from build123d import *

# Parameters (mm, degrees)
SKETCH1_W           = 11.699975178
SKETCH1_H           = 11.699996949
SKETCH1_W_2         = 11.699990436
SKETCH1_H_2         = 11.699981689
SKETCH1_W_3         = 11.699990437
SKETCH1_H_3         = 11.699975177
SKETCH1_W_4         = 11.699981689
SKETCH1_H_4         = 11.699990436
BOSS_EXTRUDE1_DEPTH = 1817.878
CUT_EXTRUDE1_REACH  = 1819.878


with BuildPart() as part:
    # Sketch1 → Boss-Extrude1 (new body)
    with BuildSketch(Plane.XY):
        Polygon((22.500515052, 22.499297556), (-22.499484399, 22.499298105), (-22.499484948, -22.500701346), (-4.249491942, -22.500701568), (-4.249491942, -22.200733242), (-4.24949208, -18.000719999), (-6.799479919, -18.000719999), (-6.799480207, -9.200732353), (-4.799480391, -7.200732362), (4.800525817, -7.200732047), (6.8005258, -9.200731855), (6.800526088, -18.000720263), (4.250507877, -18.000720263), (4.250508015, -22.200733153), (4.250508015, -22.500701672), (22.500514502, -22.500701895), (22.500514725, -4.250714302), (22.200520351, -4.250714302), (18.000507108, -4.25071444), (18.000507108, -6.800702279), (9.200519462, -6.800702567), (7.200519471, -4.800702751), (7.200519156, 4.799303458), (9.200518964, 6.79930344), (18.000507424, 6.799303729), (18.000507424, 4.249285514), (22.200520261, 4.249285652), (22.500514829, 4.249285652), align=None)
        with BuildLine():
            Line((-4.249491247, 17.999291576), (-4.249490956, 22.199304807))
            Line((-4.249490956, 22.199304807), (-3.949472548, 22.199304807))
            Line((-3.949472548, 22.199304807), (-3.481695222, 21.73152644))
            ThreePointArc((-3.481695222, 21.73152644), (-2.670636178, 21.189593132), (-1.713926324, 20.999291428))
            Line((-1.713926324, 20.999291428), (1.714975167, 20.999291428))
            ThreePointArc((1.714975167, 20.999291428), (2.671722509, 21.189608628), (3.482801459, 21.731583767))
            Line((3.482801459, 21.731583767), (3.950490798, 22.199304487))
            Line((3.950490798, 22.199304487), (4.250509108, 22.199304487))
            Line((4.250509108, 22.199304487), (4.250508817, 17.999291575))
            Line((4.250508817, 17.999291575), (6.800527063, 17.999291575))
            Line((6.800527063, 17.999291575), (6.800526453, 9.199302988))
            Line((6.800526453, 9.199302988), (4.800526064, 7.199302969))
            Line((4.800526064, 7.199302969), (-4.799479817, 7.199303635))
            Line((-4.799479817, 7.199303635), (-6.799479854, 9.199304042))
            Line((-6.799479854, 9.199304042), (-6.799479244, 17.999291576))
            Line((-6.799479244, 17.999291576), (-4.249491247, 17.999291576))
        make_face(mode=Mode.SUBTRACT)
        with BuildLine():
            Line((-22.199510888, 4.249285566), (-17.999497356, 4.249285704))
            Line((-17.999497356, 4.249285704), (-17.999497356, 6.79927354))
            Line((-17.999497356, 6.79927354), (-9.199509947, 6.799273828))
            Line((-9.199509947, 6.799273828), (-7.199509956, 4.799274012))
            Line((-7.199509956, 4.799274012), (-7.199509641, -4.800732197))
            Line((-7.199509641, -4.800732197), (-9.199509449, -6.800732179))
            Line((-9.199509449, -6.800732179), (-17.99949762, -6.800732468))
            Line((-17.99949762, -6.800732468), (-17.99949762, -4.250714253))
            Line((-17.99949762, -4.250714253), (-22.199510799, -4.250714391))
            Line((-22.199510799, -4.250714391), (-22.199510799, -3.950696126))
            Line((-22.199510799, -3.950696126), (-21.731790056, -3.48300681))
            ThreePointArc((-21.731790056, -3.48300681), (-21.189814855, -2.671927844), (-20.999497617, -1.71518046))
            Line((-20.999497617, -1.71518046), (-20.999497617, 1.713721031))
            ThreePointArc((-20.999497617, 1.713721031), (-21.189799286, 2.670430863), (-21.731732544, 3.481489907))
            Line((-21.731732544, 3.481489907), (-22.199510888, 3.949267256))
            Line((-22.199510888, 3.949267256), (-22.199510888, 4.249285566))
        make_face(mode=Mode.SUBTRACT)
        with Locations((-14.649542346, -14.650709384)):
            Rectangle(SKETCH1_W, SKETCH1_H, mode=Mode.SUBTRACT)
        with Locations((14.65050626, -14.650767962)):
            Rectangle(SKETCH1_W_2, SKETCH1_H_2, mode=Mode.SUBTRACT)
        with BuildLine():
            Line((-3.181457266, -4.596908447), (-4.595670829, -3.182694885))
            Line((-4.595670829, -3.182694885), (-3.26221457, -1.849238626))
            ThreePointArc((-3.26221457, -1.849238626), (-3.749476751, -0.00071437), (-3.26221457, 1.847809887))
            Line((-3.26221457, 1.847809887), (-4.595670829, 3.181266146))
            Line((-4.595670829, 3.181266146), (-3.181457266, 4.595479708))
            Line((-3.181457266, 4.595479708), (-1.848001007, 3.262023449))
            ThreePointArc((-1.848001007, 3.262023449), (0.000523249, 3.74928563), (1.849047505, 3.262023449))
            Line((1.849047505, 3.262023449), (3.182503764, 4.595479708))
            Line((3.182503764, 4.595479708), (4.596717327, 3.181266146))
            Line((4.596717327, 3.181266146), (3.263261068, 1.847809887))
            ThreePointArc((3.263261068, 1.847809887), (3.750523249, -0.00071437), (3.263261068, -1.849238626))
            Line((3.263261068, -1.849238626), (4.596717327, -3.182694885))
            Line((4.596717327, -3.182694885), (3.182503764, -4.596908447))
            Line((3.182503764, -4.596908447), (1.849047505, -3.263452188))
            ThreePointArc((1.849047505, -3.263452188), (0.000523249, -3.75071437), (-1.848001007, -3.263452188))
            Line((-1.848001007, -3.263452188), (-3.181457266, -4.596908447))
        make_face(mode=Mode.SUBTRACT)
        with Locations((-14.64949028, 14.649335967)):
            Rectangle(SKETCH1_W_3, SKETCH1_H_3, mode=Mode.SUBTRACT)
        with Locations((14.650561583, 14.6492839)):
            Rectangle(SKETCH1_W_4, SKETCH1_H_4, mode=Mode.SUBTRACT)
    extrude(amount=BOSS_EXTRUDE1_DEPTH)

    # Sketch1_4 → Cut-Extrude1 (cut, up to next)
    with BuildSketch(Plane.XY, mode=Mode.PRIVATE) as cut_extrude1_sk1:
        with BuildLine():
            Line((-4.249490956, 22.499297883), (-4.249490956, 22.199304807))
            Line((-4.249490956, 22.199304807), (-3.949472548, 22.199304807))
            Line((-3.949472548, 22.199304807), (-3.481695222, 21.73152644))
            ThreePointArc((-3.481695222, 21.73152644), (-2.670636178, 21.189593132), (-1.713926324, 20.999291428))
            Line((-1.713926324, 20.999291428), (1.714975167, 20.999291428))
            ThreePointArc((1.714975167, 20.999291428), (2.671722509, 21.189608628), (3.482801459, 21.731583767))
            Line((3.482801459, 21.731583767), (3.950490798, 22.199304487))
            Line((3.950490798, 22.199304487), (4.250509108, 22.199304487))
            Line((4.250509108, 22.199304487), (4.250509108, 22.499297779))
            Line((4.250509108, 22.499297779), (-4.249490956, 22.499297883))
        make_face()
    cut_extrude1_tool1 = extrude(cut_extrude1_sk1.sketch, amount=CUT_EXTRUDE1_REACH, mode=Mode.PRIVATE) & part.part
    add(cut_extrude1_tool1.solids().sort_by_distance((0.000518, 21.824215, 0))[0], mode=Mode.SUBTRACT)


solid = part.part
For this review, take the finished solid that the model builds, in its own axes (mm). Give positions to 0.01 mm unless a question says otherwise; leave off trailing zeros. Answer in a Markdown table with one row per item. Add a question column.
(1) For pin 1 (2 mm diameter, centred on x = 1.5, z = 931, fed in from +Y); pin 2 (2 mm diameter, centred on x = 2, y = -8.5, fed in from -Z); pin 3 (3 mm diameter, centred on y = 1, z = 1012, fed in from +X), all flat-tipped, find the tip position at first contact; note any pin that passes through.
(2) Wall thickness on probe 1 along Y at (x, z) = (20, 1070.5); probe 2 along Y at (x, z) = (-17, 775.5); probe 3 along X at (y, z) = (-1.5, 1654): over which ranges is each line inside the solid? List them lowest first. Write a range as [from, to].
(3) Consider section A-A on z = 1390. Give the number of separate pieces and of enclosed holes in the cut face, and give its area (3 significant figures).
Evaluation:
| question | item | result |
|---|---|---|
| 1 | pin 1 | stops at y = 7.2 |
| 1 | pin 2 | passes through |
| 1 | pin 3 | stops at x = 7.2 |
| 2 | probe 1 | y = [-22.5, -20.5], [-8.8, -4.25], [4.25, 8.8], [20.5, 22.5] |
| 2 | probe 2 | y = [-22.5, -20.5], [-8.8, -6.8], [6.8, 8.8], [20.5, 22.5] |
| 2 | probe 3 | x = [-22.5, -21], [-7.2, -3.44], [3.44, 7.2] |
| 3 | separate pieces | 1 |
| 3 | enclosed holes | 6 |
| 3 | area | 705 mm^2 |
